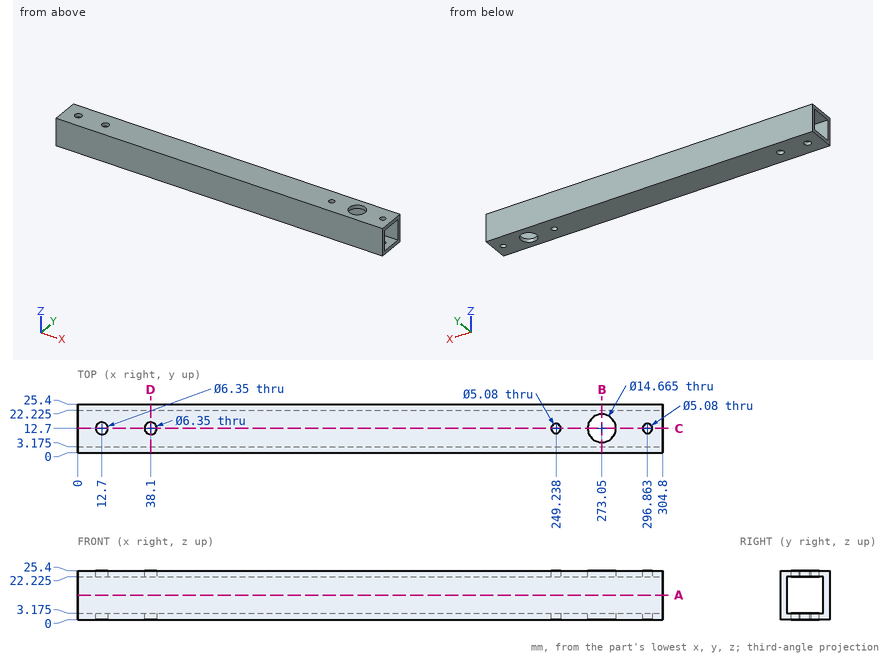
Job drawing, mm, ordinate dimensions from the low corner. One solid piece. Round coordinates to 2 decimals unless told otherwise and drop trailing zeros. Order: outer loops, then holes, each group sorted by start corner. A loop starts at its lowest first (then second) coordinate and runs counter-clockwise, first axis right, second up. Notation, with made-up numbers: M 76.25,9 L 106.25,9 A35 ccw 106.25,45 Z; hole C 45,24 d5. An arc over 180 degrees is marked long. Write each question's results on one line, items separated by ' | '. Start each with the question number.
(1) Saw through at D-D, the plane x = 38.1. Give the cut face in (y, z) (1 decimal).
(2) Saw through at B-B, the plane x = 273.05. Give the cut face in (y, z) (1 decimal).
(3) Saw through at A-A, the plane z = 12.75. Give the cut face in (x, y) (1 decimal).
(4) Saw through at C-C, the plane y = 12.7. State how many separate pieces and enclosed holes the cut face has, then the cut area to 3 significant figures.
(5) Probe probe 1 along Y at (x, z) = (38.1, 24.05) (1 decimal); probe 2 along Z at (x, y) = (41.5, 6) (1 decimal). List the from-to ranges inside material, lowest first. Write a range as from..to.
(6) Drop a flat-ended pin along its axis: pin 1 (4.5 mm diameter, centred on x = 249.24, y = 12.7, fed in from -Z). Give the stop position or say it passes through.
Established:
1) outline: M 0,0 L 9.5,0 L 9.5,3.2 L 3.2,3.2 L 3.2,22.2 L 9.5,22.2 L 9.5,25.4 L 0,25.4 Z; M 15.9,0 L 25.4,0 L 25.4,25.4 L 15.9,25.4 L 15.9,22.2 L 22.2,22.2 L 22.2,3.2 L 15.9,3.2 Z
2) outline: M 0,0 L 5.4,0 L 5.4,3.2 L 3.2,3.2 L 3.2,22.2 L 5.4,22.2 L 5.4,25.4 L 0,25.4 Z; M 20,0 L 25.4,0 L 25.4,25.4 L 20,25.4 L 20,22.2 L 22.2,22.2 L 22.2,3.2 L 20,3.2 Z
3) outline: M 0,0 L 304.8,0 L 304.8,3.2 L 0,3.2 Z; M 0,22.2 L 304.8,22.2 L 304.8,25.4 L 0,25.4 Z
4) separate pieces: 12 | enclosed holes: 0 | area: 1,700 mm^2
5) probe 1: y = 0..9.5, 15.9..25.4 | probe 2: z = 0..3.2, 22.2..25.4
6) pin 1: passes through
